Verification items for the finished model (mm, model axes). Round coordinates to 2 decimals unless told otherwise and drop trailing zeros. Write each loop counter-clockwise with the first axis right and the second up, starting at its lowest first coordinate (ties: lowest second). Pieces come first, ordered by that corner, then holes. Notation, with made-up numbers: M 80.25,2.25 L 110.25,2.25 A22 ccw 110.25,8.25 Z; hole C 12,38 d1. An arc over 180 degrees is marked long. Write each question's results on one line, items separated by ' | '.
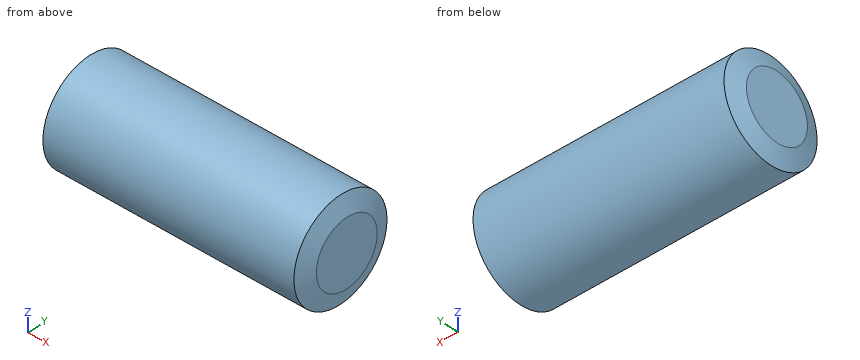
Autodesk Inventor part; units mm, degrees
ref_plane "YZ Plane" through (0, 0, 0) normal (1, 0, 0) x (0, 1, 0)
ref_plane "XZ Plane" through (0, 0, 0) normal (0, 1, 0) x (-1, 0, 0)
ref_plane "XY Plane" through (0, 0, 0) normal (0, 0, 1) x (1, 0, 0)
sketch "Base Body Sketch" plane through (0, 0, 0) normal (1, 0, 0) x (0, 1, 0)
  circle A0 centre (0, 0) radius 11.4503
  dimension "d5" = 22.9006
extrude "Base Body" add sketch "Base Body Sketch" along normal mid plane 60
sketch "Sketch5" plane through (30, 0, 0) normal (1, 0, 0) x (0, 0, -1)
  circle A0 centre (0, 0) radius 11.4503
  circle A1 centre (0, 0) radius 9.6503
  dimension "d59" = 19.3006
surface extrude "Pitch Diameter" sketch "Sketch5" against normal through all shown no curves A1
chamfer "Chamfer1" distance 1.4413 distance2 3.96 1 edges at (30, -11.4503, 0) measured on face at (20, 11.4132, -0.9214)
chamfer "Chamfer2" distance 1.4413 distance2 3.96 1 edges at (-30, -11.4503, 0) measured on face at (-20, 11.4132, -0.9214)
sketch "Tooth Sketch" plane through (0, 0, 0) normal (0, 0, 1) x (1, 0, 0)
  line L0 (0, 21.74) -> (0, 10.96)
  line L1 (-38.8672, 11.5648) -> (-37.3842, 7.4903)
  line L2 (-36.1291, 7.4903) -> (-34.6461, 11.5648)
  line L3 (-50.5346, 0) -> (-37.4554, 0)
  line L4 (-38.8672, 11.5648) -> (-36.7566, 11.5648)
  line L5 (-36.7566, 11.5648) -> (-34.6461, 11.5648)
  line L6 (-37.3842, 7.4903) -> (-36.7566, 7.4903)
  line L7 (-36.7566, 7.4903) -> (-36.1291, 7.4903)
  line L8 (-36.7566, 9.6503) -> (-35.3429, 9.6503) construction
  line L9 (-36.7566, 11.5648) -> (-36.7566, 7.4903) construction
  dimension "d24" = 110
  dimension "d25" = 36.7566
  dimension "d26" = 1.4137
  dimension "d27" = 7.4903
  dimension "d28" = 9.6503
  dimension "d29" = 11.5648
feature "Tooth" [suppressed]
pattern_circular "Tooth Pattern" [suppressed]
feature "Left Tooth" [suppressed]
pattern_circular "Left Tooth Pattern" [suppressed]
equation "\"d6\" = da_b"
equation "\"d8\" = fd_cham1"
equation "\"d9\" = 0.5 * fd_cham2"
equation "\"d10\" = fd_cham1"
equation "\"d11\" = 0.5 * fd_cham2"
equation "\"d25\" = fd_dist"
equation "\"d26\" = 0.25 * da_px"
equation "\"d27\" = 0.5 * da_df"
equation "\"d28\" = 0.5 * da_d"
equation "\"d29\" = 0.505 * da_da"
equation "\"d32\" = fd_n"
equation "\"da_rightdir\" = 0"
equation "\"d64\" = fd_n"
equation "\"d5\" = da_da"
equation "\"d59\" = da_d"
equation "\"da_aw\" = 68.15028"
equation "\"da_b\" = 60"
equation "\"da_df\" = 14.98056"
equation "\"da_da\" = 22.90056"
equation "\"fd_cham2\" = da_da - da_df"
equation "\"fd_cham1\" = 0.181985 * fd_cham2"
equation "\"da_d\" = 19.30056"
equation "\"da_px\" = 5.65487"
equation "\"da_alfat\" = 20deg"
equation "\"d49\" = da_aw"
equation "\"d79\" = da_aw"
properties part number "Worm" material "Steel, Mild"
1) Depth check by flat-ended pin: P1, Ø2, axis at x = -3, y = -3.5, coming from the +Z side; P2, Ø6, axis at y = -7.5, z = -9, coming from the -X side; P3, Ø4, axis at x = 13.5, z = -4, coming from the -Y side. Enter the tip coordinate at first touch or a pass-through.
Calculated:
P1: stops at z = 11.17 | P2: stops at x = -29.55 | P3: stops at y = -11.27
2) Sectioned sample at A-A, the plane x = -3.5. Record the cut outline in (y, z).
Calculated:
outline: C 0,0 d22.9
3) Material ranges on line 1 (Y direction, x = 8.5, z = -0.5); line 2 (Y direction, x = -7, z = -4.25); line 3 (X direction, y = 6, z = 8.75), recorded low to high. Write a range as [from, to].
Calculated:
line 1: y = [-11.44, 11.44] | line 2: y = [-10.63, 10.63] | line 3: x = [-28.86, 28.86]
